Drawing for the job (mm, zero at the part's lowest x, y, z). A direction names the side the tool comes from. Coordinates: 2 decimals unless noted, no trailing zeros. Order: outer loops, then holes, each group sorted by start corner. A loop starts at its lowest first (then second) coordinate and runs counter-clockwise, first axis right, second up.
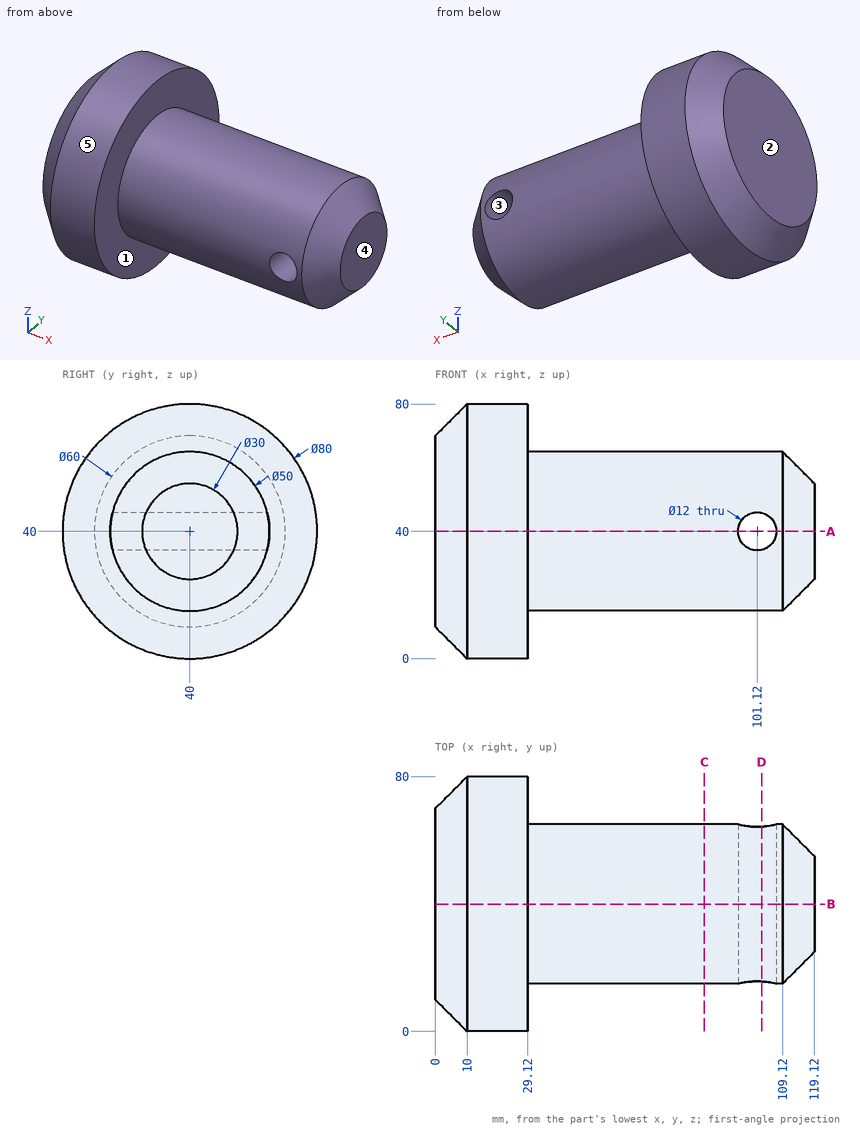
(1) Slice it at D-D, the plane x = 102.5. Give the cut face in (y, z), then the cut area to 4 significant figures.
(2) Pull direction Z, two halves, no side cores. Call the marked faces 3, 4 and 5: +Z half, -Z half, draft (parallel to the pull), parting line (faces both ways), or undercut.
(3) Tool access for the marked faces 1 and 2: list every direction of +Z, -Z, +X, -X, +Y, -Y with a clear straight run to the whole face (end or side of a thin tool).
(4) Drop flat-ended pins along their axis: pin 1 (1.5 mm diameter, centred on y = 8.5, z = 41.5, fed in from -X) (1 decimal); pin 2 (1 mm diameter, centred on x = 25, y = 56, fed in from +Z) (1 decimal); pin 3 (8 mm diameter, centred on x = 42, z = 16.5, fed in from -Y) (1 decimal). Give the stop position or say it passes through.
(5) Slice it at C-C, the plane x = 84.5. Give the cut face in (y, z).
(6) Slice it at B-B, the plane y = 40. Give the cut face in (x, z).
(7) Probe line 1 (X direction, y = 28, z = 40); line 2 (Y direction, x = 28, z = 38.5); line 3 (Z direction, x = 49, y = 28). List the from-to ranges inside material, lowest first.
(8) Slice it at A-A, the plane z = 40. Give the cut face in (x, y).
Here are the results:
1. outline: (15.69, 34.16) arc R25 ccw to (64.31, 34.16) - close; (15.69, 45.84) - (64.31, 45.84) arc R25 ccw to start
1. area: 1,385 mm2
2. face 3: undercut
2. face 4: draft
2. face 5: parting line
3. face 1: +X
3. face 2: +Z, -Z, -X, +Y, -Y
4. pin 1: stops at x = 0.8
4. pin 2: stops at z = 76.9
4. pin 3: stops at y = 24.4
5. outline: circle Ø50 at (40, 40)
6. outline: (0, 10) - (10, 0) - (29.12, 0) - (29.12, 15) - (109.12, 15) - (119.12, 25) - (119.12, 55) - (109.12, 65) - (29.12, 65) - (29.12, 80) - (10, 80) - (0, 70) - close; hole circle Ø12 at (101.12, 40)
7. line 1: x = 0 to 95.12, 107.12 to 119.12
7. line 2: y = 0.03 to 79.97
7. line 3: z = 18.07 to 61.93
8. outline: (0, 10) - (10, 0) - (29.12, 0) - (29.12, 15) - (95.12, 15) - (95.12, 65) - (29.12, 65) - (29.12, 80) - (10, 80) - (0, 70) - close; (107.12, 15) - (109.12, 15) - (119.12, 25) - (119.12, 55) - (109.12, 65) - (107.12, 65) - close
